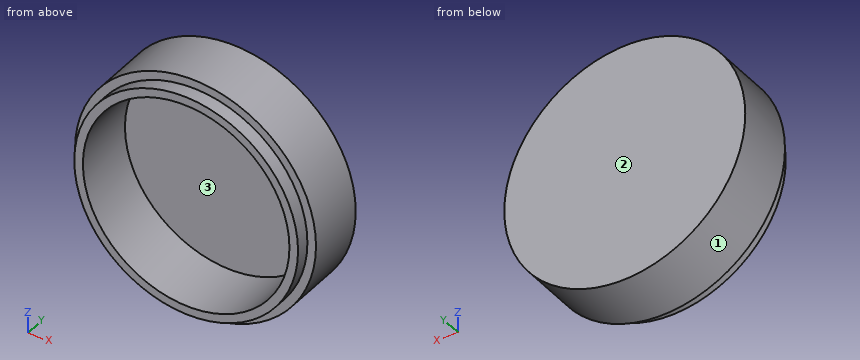
```python
from build123d import *

# Parameters (mm, degrees)
F0_R     = 35
F1_DEPTH = 21
F2_R     = 30
F3_DEPTH = 18
F4_R     = 35
F4_R_2   = 32.5
F5_DEPTH = 4


with BuildPart() as f1:
    # F0 (on Front) → F1 (new body)
    with BuildSketch(Plane.XZ):
        Circle(F0_R)
    extrude(amount=F1_DEPTH)

    # F2 (on face) → F3 (cut)
    with BuildSketch(Plane.XZ.offset(21)):
        Circle(F2_R)
    extrude(amount=-F3_DEPTH, mode=Mode.SUBTRACT)

    # F4 (on face) → F5 (cut)
    with BuildSketch(Plane.XZ.offset(21)):
        Circle(F4_R)
        Circle(F4_R_2, mode=Mode.SUBTRACT)
    extrude(amount=-F5_DEPTH, mode=Mode.SUBTRACT)


solid = f1.part
```
Design review of the part built by this model. Coordinates are the model's own, in mm. Face numbers are marked on the shaded views. Give positions to 0.01 mm unless a question says otherwise; leave off trailing zeros. Write each loop counter-clockwise with the first axis right and the second up, starting at its lowest first coordinate (ties: lowest second). Pieces come first, ordered by that corner, then holes. Notation, with made-up numbers: (80.25, 25) - (134.25, 25) arc R25 ccw to (134.25, 56) - close; hole circle Ø8 at (30.5, 60.25). An arc over 180 degrees is marked (long way). Return JSON: item names as keys, results as strings. Group by question number.
(1) Mouldability with a two-part tool opening along X and no side actions: class the marked faces 1, 2 and 3 as +X half, -X half, draft (parallel to the pull), parting line (faces both ways), or undercut.
(2) We need section B-B, the plane x = 0. Give the boundary of the cut face in (y, z), then the cut area to 3 significant figures.
(3) To check wall thickness, follow probe 1 along Z at (x, y) = (0, -15.5); probe 2 along Y at (x, z) = (23.5, 13); probe 3 along X at (y, z) = (-7, 15). State the ranges of each line that lie inside material, in increasing order.
(4) Insertion check: pin 1 (12 mm diameter, centred on x = -21.5, y = -8.5, fed in from -Z); pin 2 (2 mm diameter, centred on x = -19.5, z = 4, fed in from -Y); pin 3 (1.5 mm diameter, centred on x = 23.5, y = -5.5, fed in from -Z). Each pin has a flat end and moves straight along its axis. Give the tip position at first contact, or say it passes through.
(5) We need section C-C, the plane y = -15. Give the boundary of the cut face in (x, z).
(6) We need section A-A, the plane z = 0. Give the boundary of the cut face in (x, y), then the cut area to 3 significant figures.
Reported:
{
 "1": {"face 1": "parting line", "face 2": "draft", "face 3": "undercut"},
 "2": {"outline": "(-21, -32.5) - (-17, -32.5) - (-17, -35) - (0, -35) - (0, 35) - (-17, 35) - (-17, 32.5) - (-21, 32.5) - (-21, 30) - (-3, 30) - (-3, -30) - (-21, -30) - close", "area": "370 mm2"},
 "3": {"probe 1": "z = -35 to -30, 30 to 35", "probe 2": "y = -3 to 0", "probe 3": "x = -31.62 to -25.98, 25.98 to 31.62"},
 "4": {"pin 1": "stops at z = -31.38", "pin 2": "stops at y = -3", "pin 3": "stops at z = -26.6"},
 "5": {"outline": "circle Ø70 at (0, 0); hole circle Ø60 at (0, 0)"},
 "6": {"outline": "(-35, -17) - (-32.5, -17) - (-32.5, -21) - (-30, -21) - (-30, -3) - (30, -3) - (30, -21) - (32.5, -21) - (32.5, -17) - (35, -17) - (35, 0) - (-35, 0) - close", "area": "370 mm2"}
}
